Geometry check sheet. Reference: the model listing, model coordinates, mm. A direction names the side the tool comes from. Round coordinates to 2 decimals unless told otherwise and drop trailing zeros. Order: outer loops, then holes, each group sorted by start corner. A loop starts at its lowest first (then second) coordinate and runs counter-clockwise, first axis right, second up. Notation, with made-up numbers: M -11,2 L 40,2 A23 cw 40,14 Z; hole C 13.5,47 d9. An arc over 180 degrees is marked long. Answer as a JSON object with one key per item and string values. Group by question number.
Autodesk Inventor part; units mm, degrees
ref_plane "YZ Plane" through (0, 0, 0) normal (1, 0, 0) x (0, 1, 0)
ref_plane "XZ Plane" through (0, 0, 0) normal (0, 1, 0) x (-1, 0, 0)
ref_plane "XY Plane" through (0, 0, 0) normal (0, 0, 1) x (1, 0, 0)
sketch "Sketch1" plane through (0, 0, 0) normal (0, 1, 0) x (-1, 0, 0)
  line L0 (0, 0) -> (70, 0)
  line L1 (70, 0) -> (70, -55)
  line L2 (70, -55) -> (0, -55)
  line L3 (0, -55) -> (0, 0)
  dimension "d0" = 70
  dimension "d1" = 55
extrude "Extrusion1" add sketch "Sketch1" along normal blind 4
sketch "Sketch9" plane through (0, 4, 0) normal (0, 1, 0) x (1, 0, 0)
  line L0 (-70, 0) -> (0, 0)
  line L1 (-70, 55) -> (-70, 0)
  line L2 (-45, 0) -> (-70, 0)
  line L3 (-70, 0) -> (-70, 15)
  line L4 (-70, 15) -> (-45, 0)
  line L5 (0, 55) -> (-70, 55)
  line L6 (-45, 55) -> (-70, 55)
  line L7 (-70, 55) -> (-70, 40)
  line L8 (-70, 40) -> (-45, 55)
  dimension "d11" = 15
  dimension "d12" = 15
  dimension "d37" = 25
  dimension "d38" = 25
extrude "Extrusion4" cut sketch "Sketch9" against normal blind 4
shell "Shell1" thickness 2 removed faces 1 at (-15, 4, -18.3333)
properties part number "Foot"
1) Set-up check for faces 4 (the flat face through (-70, 2, -27)), 5 (the flat face through (-2, 3, -28)): record each of +Z, -Z, +X, -X, +Y, -Y from which the full face is reachable in a straight line by a thin tool's end or side.
2) Sectioned sample at B-B (z = -30.5). Record the boundary of the cut face in (x, y).
3) Sectioned sample at A-A (x = -15). Record the boundary of the cut face in (y, z).
4) Go/stop test with flat-tipped pins: P1, Ø2, axis at x = -58, z = -27, coming from the +Y side; P2, Ø2, axis at y = 3.5, z = -12.5, coming from the -X side. Record where each tip stops, or that it passes through.
5) Release check for a two-part mould opening along Z. For faces 1 (the flat face through (-57.675, 2.028, -47.395)), 2 (the flat face through (-56.388, 3.014, -9.165)), 3 (the flat face through (-35, 0, -27)) record: +Z half, -Z half, draft (parallel to the pull), parting line (faces both ways), or undercut.
6) Thickness scan on line 1 along X through (y, z) = (2.3, -30); line 2 along Z through (x, y) = (-5, 2.35); line 3 along Y through (x, z) = (-40.5, -41.5). Record the ranges inside material, lowest first. Write a range as [from, to].
7) Sectioned sample at C-C (y = 0.8). Record the boundary of the cut face in (x, z), then the cut area to 4 significant figures.
Final values:
{
 "1": {"face 4": "+Z, -Z, -X, +Y, -Y", "face 5": "+Y"},
 "2": {"outline": "M -70,0 L 0,0 L 0,4 L -2,4 L -2,2 L -68,2 L -68,4 L -70,4 Z"},
 "3": {"outline": "M 0,-55 L 4,-55 L 4,-53 L 2,-53 L 2,-2 L 4,-2 L 4,0 L 0,0 Z"},
 "4": {"P1": "stops at y = 2", "P2": "stops at x = -67.5"},
 "5": {"face 1": "-Z half", "face 2": "undercut", "face 3": "draft"},
 "6": {"line 1": "x = [-70, -68], [-2, 0]", "line 2": "z = [-55, -53], [-2, 0]", "line 3": "y = [0, 2]"},
 "7": {"outline": "M -70,-40 L -45,-55 L 0,-55 L 0,0 L -45,0 L -70,-15 Z", "area": "3,475 mm^2"}
}
